from build123d import *

# Parameters (mm, degrees)
F0_W     = 6
F0_H     = 6
F0_R     = 1.5
F1_DEPTH = 6
F2_R     = 1.5
F3_DEPTH = 25
F4_R     = 2.5
F5_DEPTH = 25


with BuildPart() as f1:
    # F0 (on Top) → F1 (new body)
    with BuildSketch(Plane.XY):
        Rectangle(F0_W, F0_H)
        Circle(F0_R, mode=Mode.SUBTRACT)
    extrude(amount=F1_DEPTH)

    # F2 (on face) → F3 (cut)
    with BuildSketch(Plane.YZ.offset(3)):
        with Locations((0, 3)):
            Circle(F2_R)
    extrude(amount=-F3_DEPTH, mode=Mode.SUBTRACT)

    # F4 (on face) → F5 (cut)
    with BuildSketch(Plane(origin=(0, 3, 0), x_dir=(-1, 0, 0), z_dir=(0, 1, 0))):
        with Locations((0, 3)):
            Circle(F4_R)
    extrude(amount=-F5_DEPTH, mode=Mode.SUBTRACT)


solid = f1.part
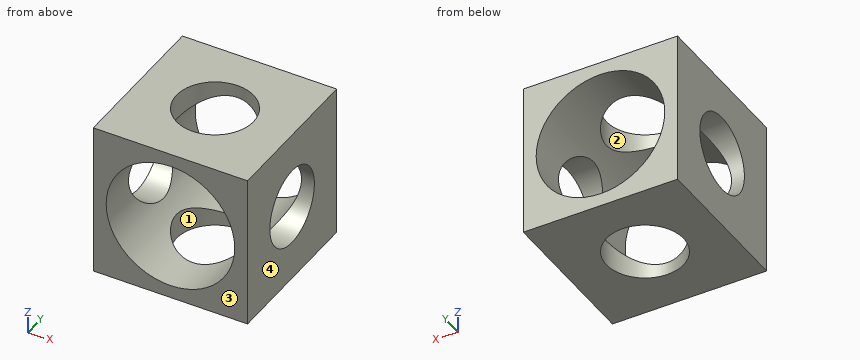
Check sheet for the modelled part. Datum: model origin and axes. Units: mm. Face numbers are marked on the shaded views. Give positions to 0.01 mm unless a question says otherwise; leave off trailing zeros. Loops run counter-clockwise (first coordinate to the right, second up) from the corner with the lowest first, then second, coordinate; pieces in that order, holes last. Notation, with made-up numbers: M -12.5,-14 L 16.5,-14 A22 ccw 16.5,13 Z; hole C 64.25,-10 d6. An arc over 180 degrees is marked long. Answer as a JSON object with one key per item and string values. Group by question number.
Q1. Cross-section at C-C on z = 3. Record the cut outline in (x, y), then the cut area to 3 significant figures.
Q2. Material ranges on line 1 along X through (y, z) = (0, 5.5); line 2 along Z through (x, y) = (2.65, 0), recorded low to high. Write a range as [from, to].
Q3. Cross-section at A-A on x = 0. Record the cut outline in (y, z).
Q4. Release check for a two-part mould opening along Y. For the marked faces 1, 2, 3 and 4 record: released by +Y, released by -Y, zero draft, split by the parting line, or undercut.
Q5. Cross-section at B-B on y = 0. Record the cut outline in (x, z), then the cut area to 3 significant figures.
Q6. Cross-section at D-D on x = 2.25. Record the cut outline in (y, z), then the cut area to 3 significant figures.
Evaluation:
{
 "1": {"outline": "M -3,-3 L -2.5,-3 L -2.5,-1.5 L -3,-1.5 Z; M -3,1.5 L -2.5,1.5 L -2.5,3 L -3,3 Z; M 2.5,-3 L 3,-3 L 3,-1.5 L 2.5,-1.5 Z; M 2.5,1.5 L 3,1.5 L 3,3 L 2.5,3 Z", "area": "3.00 mm2"},
 "2": {"line 1": "x = [-3, -1.5], [1.5, 3]", "line 2": "z = [0, 1.5], [4.5, 6]"},
 "3": {"outline": "M -3,0 L -1.5,0 L -1.5,0.5 L -3,0.5 Z; M -3,5.5 L -1.5,5.5 L -1.5,6 L -3,6 Z; M 1.5,0 L 3,0 L 3,0.5 L 1.5,0.5 Z; M 1.5,5.5 L 3,5.5 L 3,6 L 1.5,6 Z"},
 "4": {"face 1": "undercut", "face 2": "undercut", "face 3": "released by -Y", "face 4": "zero draft"},
 "5": {"outline": "M -3,0 L -1.5,0 L -1.5,1 A2.5 cw -2,1.5 L -3,1.5 Z; M -3,4.5 L -2,4.5 A2.5 cw -1.5,5 L -1.5,6 L -3,6 Z; M 1.5,0 L 3,0 L 3,1.5 L 2,1.5 A2.5 cw 1.5,1 Z; M 1.5,5 A2.5 cw 2,4.5 L 3,4.5 L 3,6 L 1.5,6 Z", "area": "8.45 mm2"},
 "6": {"outline": "M -3,0 L 3,0 L 3,1.91 L 1.03,1.91 A1.5 cw -1.03,1.91 L -3,1.91 Z; M -3,4.09 L -1.03,4.09 A1.5 cw 1.03,4.09 L 3,4.09 L 3,6 L -3,6 Z", "area": "21.8 mm2"}
}
